Verification items for the finished model (mm, model axes). Face numbers are marked on the shaded views. A direction names the side the tool comes from. Give positions to 0.01 mm unless a question says otherwise; leave off trailing zeros. Loops run counter-clockwise (first coordinate to the right, second up) from the corner with the lowest first, then second, coordinate; pieces in that order, holes last. Notation, with made-up numbers: (-9, 86.25) -> (-3, 86.25) arc R7 ccw to (-3, 96.25) -> close; hole circle Ø3 at (-23.5, 87.25). An arc over 180 degrees is marked (long way). Answer in a Markdown table with one row per item. Add a question column.
Q1. Section check B-B on y = 2. Enter the section's corners in (x, z), and give its area (3 significant figures).
Q2. Gauge pin test, flat end, axial feed: P1, Ø0.9, axis at x = 15, y = 2, coming from the -Z side. Record the tip position at first contact, or that the pin passes through.
Q3. Section check C-C on z = 9. Enter the section's corners in (x, y), and give its area (3 significant figures).
Q4. Section check A-A on z = 15. Enter the section's corners in (x, y).
Q5. Release check for a two-part mould opening along Z. For the marked faces 1, 2, 3 and 4 record: pulls with the +Z half, pulls with the -Z half, needs draft (parallel to the pull), parting line crosses it, or undercut.
Q6. Material ranges on probe 1 along X at (y, z) = (2.7, 6.75); probe 2 along Z at (x, y) = (21, 0.85); probe 3 along X at (y, z) = (2.55, 15.25), recorded low to high.
Q7. Set-up check for the marked faces 5, 6, 7 and 8: record each of +Z, -Z, +X, -X, +Y, -Y from which the full face is reachable in a straight line by a thin tool's end or side.
Q8. Section check D-D on x = 8.25. Enter the section's corners in (y, z), and give its area (3 significant figures).
```python
from build123d import *

# Parameters (mm, degrees)
EXTRUDE_1_DEPTH = 3


with BuildPart() as part:
    # 草图1 → 凸台-拉伸1 (new body)
    with BuildSketch(Plane(origin=(0, 0, 0), x_dir=(1, 0, 0), z_dir=(0, 1, 0))):
        Polygon((3, -8.25), (0, -8.25), (0, -16.5), (7.5, -16.5), (7.5, -13.5), (12.75, -13.5), (12.75, -8.25), (6, -8.25), (6, -10.75), (3, -10.75), align=None)
        Polygon((0, 0), (0, -8.25), (3, -8.25), (3, -5.75), (6, -5.75), (6, -8.25), (12.75, -8.25), (12.75, -3), (7.5, -3), (7.5, 0), align=None)
        Polygon((12.75, -3), (12.75, -8.25), (19.5, -8.25), (19.5, -5.75), (22.5, -5.75), (22.5, -8.25), (25.5, -8.25), (25.5, 0), (18, 0), (18, -3), align=None)
        Polygon((19.5, -8.25), (12.75, -8.25), (12.75, -13.5), (18, -13.5), (18, -16.5), (25.5, -16.5), (25.5, -8.25), (22.5, -8.25), (22.5, -10.75), (19.5, -10.75), align=None)
    extrude(amount=EXTRUDE_1_DEPTH)


solid = part.part
```
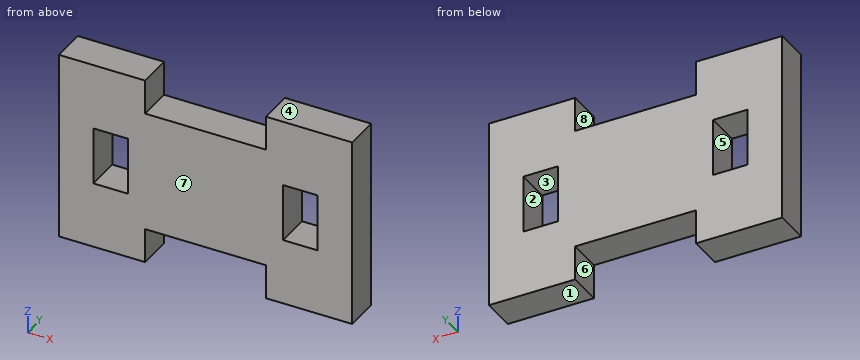
Taken from the geometry:
| question | item | result |
|---|---|---|
| 1 | outline | (0, 0) -> (7.5, 0) -> (7.5, 3) -> (18, 3) -> (18, 0) -> (25.5, 0) -> (25.5, 16.5) -> (18, 16.5) -> (18, 13.5) -> (7.5, 13.5) -> (7.5, 16.5) -> (0, 16.5) -> close; hole (3, 5.75) -> (6, 5.75) -> (6, 10.75) -> (3, 10.75) -> close; hole (19.5, 5.75) -> (22.5, 5.75) -> (22.5, 10.75) -> (19.5, 10.75) -> close |
| 1 | area | 328 mm² |
| 2 | P1 | stops at z = 3 |
| 3 | outline | (0, 0) -> (3, 0) -> (3, 3) -> (0, 3) -> close; (6, 0) -> (19.5, 0) -> (19.5, 3) -> (6, 3) -> close; (22.5, 0) -> (25.5, 0) -> (25.5, 3) -> (22.5, 3) -> close |
| 3 | area | 58.5 mm² |
| 4 | outline | (0, 0) -> (7.5, 0) -> (7.5, 3) -> (0, 3) -> close; (18, 0) -> (25.5, 0) -> (25.5, 3) -> (18, 3) -> close |
| 5 | face 1 | pulls with the -Z half |
| 5 | face 2 | undercut |
| 5 | face 3 | undercut |
| 5 | face 4 | pulls with the +Z half |
| 6 | probe 1 | x = 0 to 3, 6 to 19.5, 22.5 to 25.5 |
| 6 | probe 2 | z = 0 to 5.75, 10.75 to 16.5 |
| 6 | probe 3 | x = 0 to 7.5, 18 to 25.5 |
| 7 | face 5 | +Y, -Y |
| 7 | face 6 | -Z, +Y, -Y |
| 7 | face 7 | +Z, -Z, +X, -X, -Y |
| 7 | face 8 | +Z, +Y, -Y |
| 8 | outline | (0, 3) -> (3, 3) -> (3, 13.5) -> (0, 13.5) -> close |
| 8 | area | 31.5 mm² |
